Could you check a few things on this model? Use its own coordinates, in mm. Face numbers are marked on the shaded views. A direction names the side the tool comes from. Round coordinates to 2 decimals unless told otherwise and drop trailing zeros. Write each loop counter-clockwise with the first axis right and the second up, starting at its lowest first coordinate (ties: lowest second). Pieces come first, ordered by that corner, then holes. Notation, with made-up numbers: (83.25, 71.5) -> (120.25, 71.5) arc R26 ccw to (120.25, 97.5) -> close; hole circle Ø8 at (-6.75, 78). An arc over 180 degrees is marked (long way). Return JSON: item names as keys, results as strings.
from build123d import *

# Parameters (mm, degrees)
SKETCH2_W           = 292.1
SKETCH2_H           = 635
BOSS_EXTRUDE1_DEPTH = 190.5
CUT_EXTRUDE2_DEPTH  = 381
SHELL1_T            = -9.525
SKETCH5_W           = 292.1
SKETCH5_H           = 635
CUT_EXTRUDE3_DEPTH  = 24.892
SKETCH6_R           = 20.6375
CUT_EXTRUDE4_DEPTH  = 514.096
SKETCH10_W          = 292.1
SKETCH10_H          = 610.108
CUT_EXTRUDE7_DEPTH  = 1.693333333


with BuildPart() as part:
    # Sketch2 → Boss-Extrude1 (new body, symmetric)
    with BuildSketch(Plane(origin=(0, 0, 0), x_dir=(1, 0, 0), z_dir=(0, 1, 0))):
        Rectangle(SKETCH2_W, SKETCH2_H)
    extrude(amount=BOSS_EXTRUDE1_DEPTH, both=True)

    # Sketch4 → Cut-Extrude2 (cut)
    with BuildSketch(Plane.ZY.offset(146.05)):
        Polygon((-317.5, 190.5), (63.5, -190.5), (-317.5, -190.5), align=None)
    extrude(amount=-CUT_EXTRUDE2_DEPTH, mode=Mode.SUBTRACT)

    # Shell1
    shell1_openings = [part.faces().sort_by_distance(p)[0] for p in [
        (0, 0, 317.5),
    ]]
    offset(amount=SHELL1_T, openings=shell1_openings, kind=Kind.INTERSECTION)

    # Sketch5 → Cut-Extrude3 (cut)
    with BuildSketch(Plane(origin=(0, 190.5, 0), x_dir=(1, 0, 0), z_dir=(0, 1, 0))):
        Rectangle(SKETCH5_W, SKETCH5_H)
    extrude(amount=-CUT_EXTRUDE3_DEPTH, mode=Mode.SUBTRACT)

    # Sketch6 → Cut-Extrude4 (cut)
    with BuildSketch(Plane.ZY.offset(146.05)):
        with Locations((93.517292524, 56.961208915)):
            Circle(SKETCH6_R)
    extrude(amount=-CUT_EXTRUDE4_DEPTH, mode=Mode.SUBTRACT)

    # Sketch10 → Cut-Extrude7 (cut)
    with BuildSketch(Plane(origin=(0, 165.608, 0), x_dir=(1, 0, 0), z_dir=(0, 1, 0))):
        with Locations((0, -12.446)):
            Rectangle(SKETCH10_W, SKETCH10_H)
    extrude(amount=-CUT_EXTRUDE7_DEPTH, mode=Mode.SUBTRACT)


solid = part.part
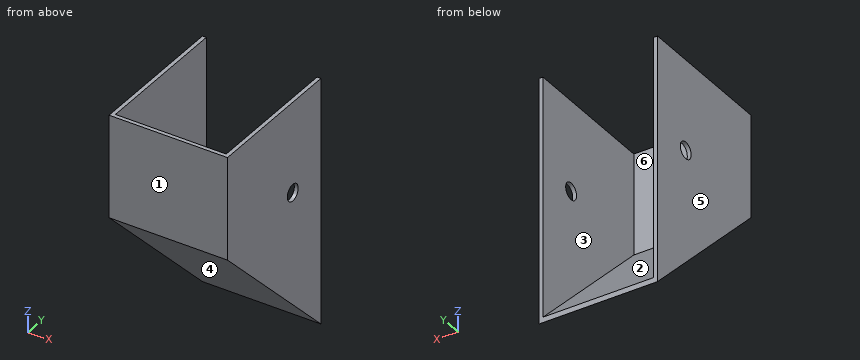
1) If I drill on probe 1 along X at (y, z) = (135.5, -90) (3 decimals); probe 2 along Y at (x, z) = (-1, 75) (3 decimals); probe 3 along Z at (x, y) = (-124, 12), over which ranges is the centre line in solid material (lowest first)? Write a range as [from, to].
Return value:
{"probe 1": "[-146.05, -136.525], [136.525, 146.05]", "probe 2": "[-190.5, -180.975]", "probe 3": "[-139, -125.53]"}
2) I want a section at D-D, the plane x = -78. Please give me the cut outline in (y, z) (3 decimals), and give its area (3 significant figures).
Return value:
{"outline": "(-190.5, 63.5) -> (163.915, -290.915) -> (163.915, -277.444) -> (-180.975, 67.445) -> (-180.975, 317.5) -> (-190.5, 317.5) -> close", "area": "7,110 mm²"}
3) I want a section at A-A, the plane z = 157. Please give me the cut outline in (x, y) (3 decimals), and give its area (3 significant figures).
Return value:
{"outline": "(-146.05, -190.5) -> (146.05, -190.5) -> (146.05, 163.915) -> (136.525, 163.915) -> (136.525, -180.975) -> (-136.525, -180.975) -> (-136.525, 163.915) -> (-146.05, 163.915) -> close", "area": "9,350 mm²"}
4) For the marked faces 1 and 2, which set-ups out of +Z, -Z, +X, -X, +Y, -Y let a thin tool reach every point of the face, with its end or its side?
Return value:
{"face 1": "+Z, -Z, +X, -X, -Y", "face 2": "+Z, +Y"}
5) I want a section at C-C, the plane y = -66.5. Please give me the cut outline in (x, z) (3 decimals).
Return value:
{"outline": "(-146.05, -60.5) -> (146.05, -60.5) -> (146.05, 317.5) -> (136.525, 317.5) -> (136.525, -47.03) -> (-136.525, -47.03) -> (-136.525, 317.5) -> (-146.05, 317.5) -> close"}
6) Will these pins go through, and if not, where does the flat tip stop? pin 1 Ø2 at (x, z) = (-29.5, -150) entering from -Y; pin 2 Ø4 at (x, z) = (86, -4) entering from -Y; pin 3 Ø6 at (x, z) = (59, -170.5) entering from +Y.
Return value:
{"pin 1": "y = 22", "pin 2": "y = -125", "pin 3": "y = 59.97"}
7) I want a section at B-B, the plane z = 82.5. Please give me the cut outline in (x, y) (3 decimals), and give its area (3 significant figures).
Return value:
{"outline": "(-146.05, -190.5) -> (146.05, -190.5) -> (146.05, 39.511) -> (136.525, 39.511) -> (136.525, -180.975) -> (-136.525, -180.975) -> (-136.525, 39.511) -> (-146.05, 39.511) -> close; (-146.05, 74.412) -> (-136.525, 74.412) -> (-136.525, 163.915) -> (-146.05, 163.915) -> close; (136.525, 74.412) -> (146.05, 74.412) -> (146.05, 163.915) -> (136.525, 163.915) -> close", "area": "8,690 mm²"}
8) Thinking about a two-plate mould opening in X: for the marked faces 3, 4, 5 and 6, which applies, pulls with the +X half, pulls with the -X half, needs draft (parallel to the pull), parting line crosses it, or undercut?
Return value:
{"face 3": "undercut", "face 4": "needs draft", "face 5": "pulls with the -X half", "face 6": "undercut"}
